The model under review builds one solid part; all positions refer to its coordinate system, in mm. A direction names the side the tool comes from. Round coordinates to 2 decimals unless told otherwise and drop trailing zeros. Loops run counter-clockwise (first coordinate to the right, second up) from the corner with the lowest first, then second, coordinate; pieces in that order, holes last. Notation, with made-up numbers: M 76.5,-37.75 L 125.5,-37.75 A27 cw 125.5,-18.75 Z; hole C 77,37.5 d10. An arc over 180 degrees is marked long. Return JSON: item names as keys, results as strings. Group by question number.
Q1. Consider section B-B (x = 118.5). State the section outline as (y, z) points, and give its area (3 significant figures).
Q2. Clearance check with flat-ended pins moving along their axes: pin 1 Ø2 at (x, z) = (71.5, 89) entering from -Y; pin 2 Ø2 at (y, z) = (-55.5, 149.5) entering from -X; pin 3 Ø18.5 at (x, z) = (194, 149) entering from -Y. State where each tip first meets the part, or that it passes through.
Q3. Draft analysis for pull direction X (two halves, no side actions). For faces 1 (the face through (230, 1, 81)), 2 (the face through (192, -32, 104)), 3 (the face through (225.944, 67.585, 153.704)), state which applies: pulls with the +X half, pulls with the -X half, needs draft (parallel to the pull), parting line crosses it, or undercut.
Q4. Consider section D-D (x = -17.5). State the section outline as (y, z) points.
Q5. Consider section A-A (x = 60). State the section outline as (y, z) points.
Q6. For faces 4 (the face through (188, -41, 77.5)), 5 (the face through (192.26, -0.03, 148.66)), 6 (the face through (192.74, -0.03, 11.66)), list the 3-axis set-ups (+Z, -Z, +X, -X, +Y, -Y) from which the entire face can be reached by the end or side of a thin tool; tool diameter is ignored.
Q7. Consider section C-C (x = 187.5). State the section outline as (y, z) points, and give its area (3 significant figures).
Q8. To check wall thickness, follow line 1 along X through (y, z) = (-15.5, 142.5); line 2 along Z through (x, y) = (197.5, -33.5); line 3 along X through (y, z) = (-24.5, 37.5). State the ranges of each line that lie inside material, in increasing order.
from build123d import *

# Parameters (mm, degrees)
BOSS_EXTRU_1_DEPTH           = 160
ESQUISSE3_R                  = 12.5
BOSS_EXTRU_3_DEPTH           = 70
CHANFREIN9_SIZE              = 20
BOSS_EXTRU_4_DEPTH           = 35
BOSS_EXTRU_5_DEPTH           = 2.5
R_P_TITION_START             = 77.5
R_P_TITION_CIRCULAIRE1_DEPTH = 5
BOSS_EXTRU_6_START           = -32
BOSS_EXTRU_6_DEPTH           = 2
R_P_TITION_START_2           = -2
R_P_TITION_CIRCULAIRE2_DEPTH = 4
ESQUISSE10_R                 = 100
BOSS_EXTRU_7_DEPTH           = 20
CONG_3_R                     = 12


# Read off the part's stored shape, not the designer's step: Répétition circulaire1, Répétition circulaire2
with BuildPart() as part:
    # Esquisse1 → Boss.-Extru.1 (new body)
    with BuildSketch(Plane.XY):
        Polygon((0, -47.5), (0, 47.5), (175, 55), (175, -55), align=None)
    extrude(amount=BOSS_EXTRU_1_DEPTH)

    # Esquisse3 → Boss.-Extru.3 (add)
    with BuildSketch(Plane.ZY):
        with Locations(Location((80, 0, 0), (0, 0, 180))):
            Circle(ESQUISSE3_R)
    extrude(amount=BOSS_EXTRU_3_DEPTH)

    # Chanfrein9
    chanfrein9_edges = [part.edges().sort_by_distance(p)[0] for p in [
        (87.5, -51.25, 160),
        (87.5, 51.25, 160),
        (87.5, -51.25, 0),
        (87.5, 51.25, 0),
    ]]
    chamfer(chanfrein9_edges, length=CHANFREIN9_SIZE)

    # Esquisse4 → Boss.-Extru.4 (add)
    with BuildSketch(Plane(origin=(175, 0, 0), x_dir=(0, 0, -1), z_dir=(1, 0, 0))):
        Polygon((-127, 32), (-33, 32), (-23, 22), (-23, -22), (-33, -32), (-127, -32), (-137, -22), (-137, 22), align=None)
    extrude(amount=BOSS_EXTRU_4_DEPTH)

    # Esquisse5 → Boss.-Extru.5 (add, symmetric)
    with BuildSketch(Plane.XY.offset(80)):
        Polygon((175, 55), (210, 32), (175, 32), align=None)
    extrude(amount=BOSS_EXTRU_5_DEPTH, both=True)

    # Répétition circulaire1 outline → Répétition circulaire1 (add)
    with BuildSketch(Plane.XY.offset(R_P_TITION_START)):
        Polygon((175, -32), (175, -55), (210, -32), align=None)
    extrude(amount=R_P_TITION_CIRCULAIRE1_DEPTH)

    # Esquisse8 → Boss.-Extru.6 (add, symmetric)
    with BuildSketch(Plane.XZ.offset(32).offset(BOSS_EXTRU_6_START)):
        Polygon((175, 160), (210, 137), (175, 137), align=None)
    extrude(amount=BOSS_EXTRU_6_DEPTH, both=True)

    # Répétition circulaire2 outline → Répétition circulaire2 (add)
    with BuildSketch(Plane(origin=(0, 0, 0), x_dir=(1, 0, 0), z_dir=(0, 1, 0)).offset(R_P_TITION_START_2)):
        Polygon((175, -23), (210, -23), (175, 0), align=None)
    extrude(amount=R_P_TITION_CIRCULAIRE2_DEPTH)

    # Esquisse10 → Boss.-Extru.7 (add)
    with BuildSketch(Plane(origin=(210, 0, 0), x_dir=(0, 0, -1), z_dir=(1, 0, 0))):
        with Locations((-80, 0)):
            Circle(ESQUISSE10_R)
    extrude(amount=BOSS_EXTRU_7_DEPTH)

    # Congé3
    cong_3_edges = [part.edges().sort_by_distance(p)[0] for p in [
        (210, 0, 180),
    ]]
    fillet(cong_3_edges, radius=CONG_3_R)


solid = part.part
Values:
{
 "1": {"outline": "M -52.58,20 L -32.56,0 L 32.56,0 L 52.58,20 L 52.58,140 L 32.56,160 L -32.56,160 L -52.58,140 Z", "area": "16,000 mm2"},
 "2": {"pin 1": "stops at y = -50.61", "pin 2": "stops at x = 210", "pin 3": "stops at y = -2"},
 "3": {"face 1": "pulls with the +X half", "face 2": "undercut", "face 3": "needs draft"},
 "4": {"outline": "C 0,80 d25"},
 "5": {"outline": "M -50.07,20 L -30.05,0 L 30.05,0 L 50.07,20 L 50.07,140 L 30.05,160 L -30.05,160 L -50.07,140 Z"},
 "6": {"face 4": "-Z, -Y", "face 5": "+Z, +Y, -Y", "face 6": "-Z, +Y, -Y"},
 "7": {"outline": "M -46.79,77.5 L -32,77.5 L -32,33 L -22,23 L -2,23 L -2,8.21 L 2,8.21 L 2,23 L 22,23 L 32,33 L 32,77.5 L 46.79,77.5 L 46.79,82.5 L 32,82.5 L 32,127 L 22,137 L 2,137 L 2,151.79 L -2,151.79 L -2,137 L -22,137 L -32,127 L -32,82.5 L -46.79,82.5 Z", "area": "7,360 mm2"},
 "8": {"line 1": "x = 0 to 175, 210 to 230", "line 2": "z = 77.5 to 82.5", "line 3": "x = 0 to 230"}
}
